Can you work these out from the model? Positions are in its coordinate system, mm. A direction names the side the tool comes from. Give positions to 0.01 mm unless a question says otherwise; leave off trailing zeros. Order: outer loops, then holes, each group sorted by start corner. A loop starts at its lowest first (then second) coordinate and runs counter-clockwise, first axis right, second up. Notation, with made-up numbers: (51, 88) -> (76, 88) arc R34 ccw to (76, 123) -> close; hole circle Ø4 at (58.25, 66.5). An arc over 180 degrees is marked (long way). Answer as a JSON object with one key per item and string values.
```python
from build123d import *

# Parameters (mm, degrees)
F1_DEPTH = 3
F2_D     = 4.5
F3_R     = 5
F4_D     = 3.4
F6_D     = 3.4
F5_W     = 5.5
F5_H     = 13.5
F7_DEPTH = 25


# Not quite as in the source:
# - a feature names something its author has since deleted; it is built from what else it names


with BuildPart() as f1:
    # F0 (on Top) → F1 (new body)
    with BuildSketch(Plane.XY):
        Polygon((-35.8541943133, -51.5685416758), (24.4538411498, -51.5685416758), (24.4538411498, 52.9103763402), (-117.0655786991, 52.9103763402), (-117.0655786991, -14.937300235), (-35.8541943133, -14.937300235), align=None)
    extrude(amount=F1_DEPTH)

    # F2 (through all)
    with Locations(Plane(origin=(0, 0, 0), x_dir=(1, 0, 0), z_dir=(0, 0, -1))):
        with Locations((-21.5, -46.5), (21.5, -46.5), (21.5, 46.5), (-21.5, 46.5)):
            Hole(F2_D / 2)

    # F3
    f3_edges = [f1.edges().sort_by_distance(p)[0] for p in [
        (-117.065579, 52.910376, 1.5),
        (24.453841, 52.910376, 1.5),
        (24.453841, -51.568542, 1.5),
        (-35.854194, -14.9373, 1.5),
        (-35.854194, -51.568542, 1.5),
        (-117.065579, -14.9373, 1.5),
    ]]
    fillet(f3_edges, radius=F3_R)

    # F4 (through all)
    with Locations(Plane(origin=(0, 0, 0), x_dir=(1, 0, 0), z_dir=(0, 0, -1))):
        with Locations((-31.5, -46.5), (11.5, -46.5), (11.5, 4.5), (-31.5, 4.5)):
            Hole(F4_D / 2)

    # F6 (through all)
    with Locations(Plane.XY.offset(3)):
        with Locations((-59.8872532725, 3.0199595654), (-59.8872532725, 19.9299595654), (-108.7842532725, -10.8700404346)):
            Hole(F6_D / 2)

    # F5 (on face) → F7 (cut)
    with BuildSketch(Plane.XY.offset(3)):
        with Locations((-59.5872532725, 36.6799595654)):
            Rectangle(F5_W, F5_H)
    extrude(amount=-F7_DEPTH, mode=Mode.SUBTRACT)


solid = f1.part
```
1. If we section it at A-A on y = 46.5: Please give me the cut outline in (x, z), then the cut area to 3 significant figures.
Worked answers:
{"outline": "(-117.07, 0) -> (-33.2, 0) -> (-33.2, 3) -> (-117.07, 3) -> close; (-29.8, 0) -> (-23.75, 0) -> (-23.75, 3) -> (-29.8, 3) -> close; (-19.25, 0) -> (9.8, 0) -> (9.8, 3) -> (-19.25, 3) -> close; (13.2, 0) -> (19.25, 0) -> (19.25, 3) -> (13.2, 3) -> close; (23.75, 0) -> (24.45, 0) -> (24.45, 3) -> (23.75, 3) -> close", "area": "377 mm²"}
2. If we section it at C-C on z = 1.45: Count the separate pieces of the cut face and the enclosed holes in it, then the cut area to 3 significant figures.
Worked answers:
{"separate pieces": "1", "enclosed holes": "12", "area": "11,600 mm²"}
3. Please list where these lines run through material, in increasing order: L1, parallel to X at y = 46.5, z = 0.75; L2, parallel to Y at x = -21.5, z = 1.45; L3, parallel to Y at x = 11.5, z = 2.
Worked answers:
{"L1": "-117.07 to -33.2, -29.8 to -23.75, -19.25 to 9.8, 13.2 to 19.25, 23.75 to 24.45", "L2": "-51.57 to -48.75, -44.25 to 44.25, 48.75 to 52.91", "L3": "-51.57 to -6.2, -2.8 to 44.8, 48.2 to 52.91"}
4. If we section it at B-B on x = 11.5: Please give me the cut outline in (y, z), then the cut area to 3 significant figures.
Worked answers:
{"outline": "(-51.57, 0) -> (-6.2, 0) -> (-6.2, 3) -> (-51.57, 3) -> close; (-2.8, 0) -> (44.8, 0) -> (44.8, 3) -> (-2.8, 3) -> close; (48.2, 0) -> (52.91, 0) -> (52.91, 3) -> (48.2, 3) -> close", "area": "293 mm²"}
5. Will these pins go through, and if not, where does the flat tip stop? pin 1 Ø4 at (x, y) = (21.5, -46.5) entering from +Z; pin 2 Ø1.5 at (x, z) = (-60, 2) entering from -Y.
Worked answers:
{"pin 1": "through", "pin 2": "y = -14.94"}
6. For faces 5 (the face through (-62.337, 37, 2)), 6 (the face through (-115.562, 51.485, 1.521)), which set-ups out of +Z, -Z, +X, -X, +Y, -Y let a thin tool reach every point of the face, with its end or its side?
Worked answers:
{"face 5": "+Z, -Z", "face 6": "+Z, -Z, -X, +Y"}
7. If we mould it in two halves opening along X, with no side actions, what happens to faces 1 (the face through (-32, 13, 0)), 2 (the face through (-35.854, -33, 1)), 3 (the face through (-61.51, 3.53, 1.48)), 4 (the face through (-109.7, -9.44, 1.48))? For each: +X half, -X half, draft (parallel to the pull), parting line (faces both ways), or undercut.
Worked answers:
{"face 1": "draft", "face 2": "-X half", "face 3": "undercut", "face 4": "undercut"}
8. If we section it at D-D on y = -4.5: Please give me the cut outline in (x, z), then the cut area to 3 significant figures.
Worked answers:
{"outline": "(-117.07, 0) -> (-33.2, 0) -> (-33.2, 3) -> (-117.07, 3) -> close; (-29.8, 0) -> (9.8, 0) -> (9.8, 3) -> (-29.8, 3) -> close; (13.2, 0) -> (24.45, 0) -> (24.45, 3) -> (13.2, 3) -> close", "area": "404 mm²"}
